Geometry: final body of the model. Coordinates: model frame, mm. A direction names the side the tool comes from. Give positions to 0.01 mm unless a question says otherwise; leave off trailing zeros. Loops run counter-clockwise (first coordinate to the right, second up) from the corner with the lowest first, then second, coordinate; pieces in that order, holes last.
1. Section B-B, the plane x = 150. Output: boundary loops of the cut face in (y, z), then the cut area to 3 significant figures.
2. Draft query along Z for faces 3 (the face through (-3, 18, 45)), 4 (the face through (-3, 0, -11)), 5 (the face through (-140.763, 29.091, 3.83)). Return one class per face: +Z half, -Z half, draft (parallel to the pull), parting line (faces both ways), or undercut.
3. Access query for faces 1 (the face through (-3, 18, -45)), 2 (the face through (50, 29, 0)). Directions: +Z, -Z, +X, -X, +Y, -Y. A direction counts if a zero-diameter tool reaches every point of the face in a straight line with its end or side. Return the directions, or none.
4. Section A-A, the plane y = 29.5. Output: boundary loops of the cut face in (x, z), then the cut area to 3 significant figures.
5. Section D-D, the plane z = -37.5. Output: boundary loops of the cut face in (x, y).
6. First-contact query: P1, Ø15.5, axis at x = -60, z = 0, coming from the -Y side; P2, Ø12, axis at x = 150, z = 0, coming from the +Y side; P3, Ø16, axis at x = -60, z = 0, coming from the +Y side. Flat tips, straight axial feed; report the tip coordinate or a pass-through.
7. Section C-C, the plane y = 6. Output: boundary loops of the cut face in (x, z), then the cut area to 3 significant figures.
8. Material intervals for line 1 along X through (y, z) = (23, 4); line 2 along Z through (x, y) = (60, 26); line 3 along X through (y, z) = (33, 24), sorted ascending.
from build123d import *

# Parameters (mm, degrees)
SKETCH_1_W                          = 370
SKETCH_1_H                          = 90
EXTRUDE_1_DEPTH                     = 35.5
SKETCH_2_W                          = 25
SKETCH_2_H                          = 90
CUT_EXTRUDE_1_DEPTH                 = 13
HOLE_WIZARD_M4_1_D                  = 13.5
HOLE_WIZARD_M4_1_CBORE_D            = 20
HOLE_WIZARD_M4_1_CBORE_DEPTH        = 13
PATTERN_LINEAR_1_COUNT              = 2
PATTERN_LINEAR_1_PITCH              = 90
PATTERN_LINEAR_2_COPY_1_D           = 13.5
PATTERN_LINEAR_2_COPY_1_CBORE_D     = 20
PATTERN_LINEAR_2_COPY_1_CBORE_DEPTH = 13
PATTERN_LINEAR_3_COPY_1_D           = 13.5
PATTERN_LINEAR_3_COPY_1_CBORE_D     = 20
PATTERN_LINEAR_3_COPY_1_CBORE_DEPTH = 13
PATTERN_LINEAR_3_COPY_2_D           = 13.5
PATTERN_LINEAR_3_COPY_2_CBORE_D     = 20
PATTERN_LINEAR_3_COPY_2_CBORE_DEPTH = 13
HOLE_WIZARD_M4_2_D                  = 13.5
HOLE_WIZARD_M4_2_CBORE_D            = 20
HOLE_WIZARD_M4_2_CBORE_DEPTH        = 13


with BuildPart() as part:
    # 草图1 → 凸台-拉伸1 (new body)
    with BuildSketch(Plane(origin=(0, 0, 0), x_dir=(1, 0, 0), z_dir=(0, 1, 0))):
        Rectangle(SKETCH_1_W, SKETCH_1_H)
    extrude(amount=EXTRUDE_1_DEPTH)

    # 草图2 → 切除-拉伸1 (cut)
    with BuildSketch(Plane(origin=(0, 35.5, 0), x_dir=(1, 0, 0), z_dir=(0, 1, 0))):
        Rectangle(SKETCH_2_W, SKETCH_2_H)
    extrude(amount=-CUT_EXTRUDE_1_DEPTH, mode=Mode.SUBTRACT)

    # M4 六角头螺栓的柱形沉头孔1 (through all)
    with Locations(Plane(origin=(0, 35.5, 0), x_dir=(1, 0, 0), z_dir=(0, 1, 0))):
        with Locations((-150, 0)):
            hole_wizard_m4_1 = CounterBoreHole(HOLE_WIZARD_M4_1_D / 2, HOLE_WIZARD_M4_1_CBORE_D / 2, HOLE_WIZARD_M4_1_CBORE_DEPTH)

    # 阵列(线性)1: M4 六角头螺栓的柱形沉头孔1 ×2
    with Locations(*[(i * PATTERN_LINEAR_1_PITCH, 0, 0) for i in range(1, PATTERN_LINEAR_1_COUNT)]):
        add(hole_wizard_m4_1, mode=Mode.SUBTRACT)

    # 阵列(线性)2 copy 1 (through all)
    with Locations(Plane(origin=(210, 35.5, 0), x_dir=(1, 0, 0), z_dir=(0, 1, 0))):
        with Locations((-150, 0)):
            CounterBoreHole(PATTERN_LINEAR_2_COPY_1_D / 2, PATTERN_LINEAR_2_COPY_1_CBORE_D / 2, PATTERN_LINEAR_2_COPY_1_CBORE_DEPTH)

    # 阵列(线性)3 copy 1 (through all)
    with Locations(Plane(origin=(300, 35.5, 0), x_dir=(1, 0, 0), z_dir=(0, 1, 0))):
        with Locations((-150, 0)):
            CounterBoreHole(PATTERN_LINEAR_3_COPY_1_D / 2, PATTERN_LINEAR_3_COPY_1_CBORE_D / 2, PATTERN_LINEAR_3_COPY_1_CBORE_DEPTH)

    # 阵列(线性)3 copy 2 (through all)
    with Locations(Plane(origin=(90, 35.5, 0), x_dir=(1, 0, 0), z_dir=(0, 1, 0))):
        with Locations((-150, 0)):
            CounterBoreHole(PATTERN_LINEAR_3_COPY_2_D / 2, PATTERN_LINEAR_3_COPY_2_CBORE_D / 2, PATTERN_LINEAR_3_COPY_2_CBORE_DEPTH)

    # M4 六角头螺栓的柱形沉头孔2 (through all)
    with Locations(Plane(origin=(0, 22.5, 0), x_dir=(1, 0, 0), z_dir=(0, 1, 0))):
        with Locations((0, 0)):
            CounterBoreHole(HOLE_WIZARD_M4_2_D / 2, HOLE_WIZARD_M4_2_CBORE_D / 2, HOLE_WIZARD_M4_2_CBORE_DEPTH)


solid = part.part
Answers below:
1. outline: (0, -45) - (35.5, -45) - (35.5, -10) - (22.5, -10) - (22.5, -6.75) - (0, -6.75) - close; (0, 6.75) - (22.5, 6.75) - (22.5, 10) - (35.5, 10) - (35.5, 45) - (0, 45) - close
1. area: 2,630 mm2
2. face 3: +Z half
2. face 4: draft
2. face 5: undercut
3. face 1: -Z, +X, -X, +Y, -Y
3. face 2: +Y
4. outline: (-185, -45) - (-12.5, -45) - (-12.5, 45) - (-185, 45) - close; (12.5, -45) - (185, -45) - (185, 45) - (12.5, 45) - close; hole circle Ø20 at (-150, 0); hole circle Ø20 at (-60, 0); hole circle Ø20 at (60, 0); hole circle Ø20 at (150, 0)
4. area: 29,800 mm2
5. outline: (-185, 0) - (185, 0) - (185, 35.5) - (12.5, 35.5) - (12.5, 22.5) - (-12.5, 22.5) - (-12.5, 35.5) - (-185, 35.5) - close
6. P1: stops at y = 0
6. P2: passes through
6. P3: stops at y = 22.5
7. outline: (-185, -45) - (185, -45) - (185, 45) - (-185, 45) - close; hole circle Ø13.5 at (-150, 0); hole circle Ø13.5 at (-60, 0); hole circle Ø13.5 at (0, 0); hole circle Ø13.5 at (60, 0); hole circle Ø13.5 at (150, 0)
7. area: 32,600 mm2
8. line 1: x = -185 to -159.17, -140.83 to -69.17, -50.83 to -12.5, 12.5 to 50.83, 69.17 to 140.83, 159.17 to 185
8. line 2: z = -45 to -10, 10 to 45
8. line 3: x = -185 to -12.5, 12.5 to 185
